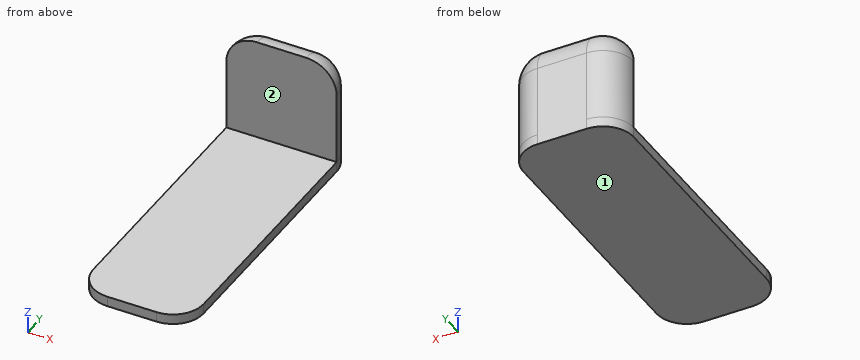
from build123d import *

# Parameters (mm, degrees)
F0_W     = 54
F0_H     = 150
F1_DEPTH = 50
F2_R     = 15
F3_R     = 15
F5_DEPTH = 5
F6_W     = 121.107407
F6_H     = 159.268379
F7_DEPTH = 50.001


with BuildPart() as f1:
    # F0 (on Top) → F1 (new body)
    with BuildSketch(Plane.XY):
        Rectangle(F0_W, F0_H)
    extrude(amount=F1_DEPTH)

    # F2
    f2_edges = [f1.edges().sort_by_distance(p)[0] for p in [
        (27, -75, 25),
        (-27, -75, 25),
        (27, 75, 25),
        (-27, 75, 25),
    ]]
    fillet(f2_edges, radius=F2_R)

    # F3
    f3_edges = [f1.edges().sort_by_distance(p)[0] for p in [
        (-27, 0, 50),
    ]]
    fillet(f3_edges, radius=F3_R)

    # F4 (on face) → F5 (join)
    with BuildSketch(Plane(origin=(0, 0, 0), x_dir=(1, 0, 0), z_dir=(0, 0, -1))):
        with BuildLine():
            ThreePointArc((12, -75), (22.606602, -70.606602), (27, -60))
            Line((27, -60), (27, 60))
            ThreePointArc((27, 60), (22.606602, 70.606602), (12, 75))
            Line((12, 75), (-12, 75))
            ThreePointArc((-12, 75), (-22.606602, 70.606602), (-27, 60))
            Line((-27, 60), (-27, -60))
            ThreePointArc((-27, -60), (-22.606602, -70.606602), (-12, -75))
            Line((-12, -75), (12, -75))
        make_face()
    extrude(amount=F5_DEPTH)

    # F6 (on Top) → F7 (cut, through all)
    with BuildSketch(Plane.XY):
        with Locations((-1.455303, -19.634189)):
            Rectangle(F6_W, F6_H)
    extrude(amount=F7_DEPTH, mode=Mode.SUBTRACT)


solid = f1.part
Input: part model. Units: mm. Frame: model coordinates. Face numbers are marked on the shaded views. A direction names the side the tool comes from. Give positions to 0.01 mm unless a question says otherwise; leave off trailing zeros. Loops run counter-clockwise (first coordinate to the right, second up) from the corner with the lowest first, then second, coordinate; pieces in that order, holes last. Notation, with made-up numbers: M -3.5,28.25 L 34.5,28.25 A21 ccw 34.5,50.25 Z; hole C 64,-38 d8. An arc over 180 degrees is marked long. Use one line per item in the form item = value.
1. Section query A-A, the plane x = 3.5. Return the cut outline in (y, z).
Numbers:
outline = M -75,-5 L 75,-5 L 75,35 A15 ccw 60,50 L 60,0 L -75,0 Z
2. First-contact query: pin 1 (1 mm diameter, centred on x = -19, y = 52, fed in from +Z); pin 2 (8 mm diameter, centred on x = -13, z = 16, fed in from -Y); pin 3 (1.5 mm diameter, centred on x = -13, z = 38.5, fed in from +Y). Flat tips, straight axial feed; report the tip coordinate or a pass-through.
Numbers:
pin_1 = 0
pin_2 = 60
pin_3 = 74.72
3. Section query C-C, the plane x = -24. Return the cut outline in (y, z).
Numbers:
outline = M -69,-5 L 69,-5 L 69,35 A9 ccw 60,44 L 60,0 L -69,0 Z
4. Line query: L1, parallel to Z at x = -18, y = -40; L2, parallel to Y at x = -10.5, z = 23; L3, parallel to Y at x = -22.5, z = 10. Output: solid intervals per line, ascending.
Numbers:
L1 = -5 to 0
L2 = 60 to 75
L3 = 60 to 70.71
5. Reachability of the marked faces 1 and 2 from +Z, -Z, +X, -X, +Y, -Y: full face, straight path, thin tool, end or side. Return the list, or none.
Numbers:
face_1 = -Z, +X, -X, +Y, -Y
face_2 = +Z, +X, -X, -Y
6. Section query D-D, the plane z = 20.5. Return the cut outline in (x, y), and give its area (3 significant figures).
Numbers:
outline = M -27,60 L 27,60 A15 ccw 12,75 L -12,75 A15 ccw Z
area = 713 mm²
7. Section query B-B, the plane y = 27.5. Return the cut outline in (x, z), and give its area (3 significant figures).
Numbers:
outline = M -27,-5 L 27,-5 L 27,0 L -27,0 Z
area = 270 mm²
